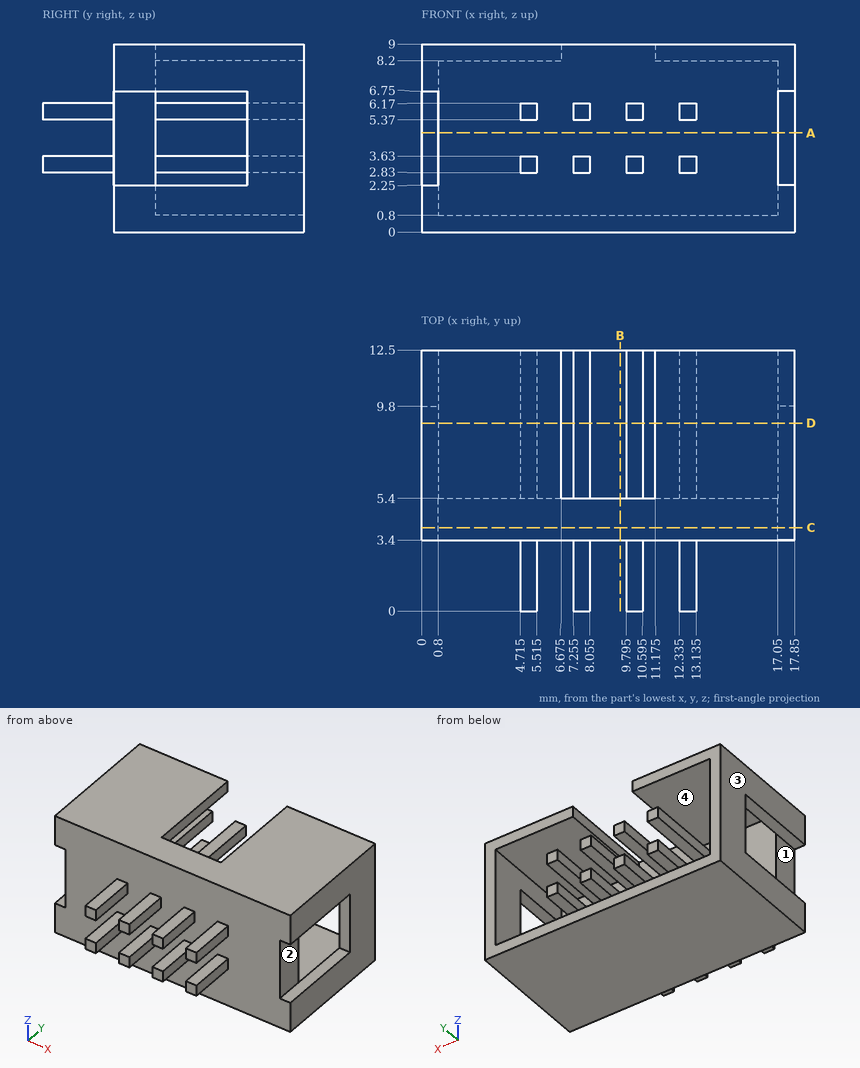
Geometry check sheet. Reference: drawing and pictorial views, mm from the part's lowest x, y, z. A direction names the side the tool comes from. Give positions to 0.01 mm unless a question says otherwise; leave off trailing zeros. Write each loop counter-clockwise with the first axis right and the second up, starting at its lowest first coordinate (ties: lowest second). Pieces come first, ordered by that corner, then holes.
Item 1: Cross-section at C-C (y = 4). Enter the section's corners in (x, z), and give its area (3 significant figures).
Item 2: Access from +Z, -Z, +X, -X, +Y, -Y to the whole of each face (thin tool, end or side, straight path). Record for the marked faces 1, 2, 3 and 4.
Item 3: Cross-section at D-D (y = 9). Count the separate pieces of the cut face and the enclosed holes in it, and give its area (3 significant figures).
Item 4: Cross-section at B-B (x = 9.5). Enter the section's corners in (y, z), and give its area (3 significant figures).
Item 5: Cross-section at A-A (z = 4.75). Enter the section's corners in (x, y), and give its area (3 significant figures).
Item 6: Scan lines: L1, parallel to Z at x = 12.5, y = 11.5; L2, parallel to X at y = 11, z = 3 (3 decimals); L3, parallel to X at y = 6, z = 1.75. Record each from-to range of solid material in increasing order.
Item 7: Gauge pin test, flat ends, axial feed: pin 1 (1 mm diameter, centred on x = 7.5, z = 2, fed in from +Y); pin 2 (0.9 mm diameter, centred on x = 5, y = 1.5, fed in from -Z); pin 3 (0.6 mm diameter, centred on y = 2, z = 6, fed in from +X) (3 decimals). Record the tip position at first contact, or that the pin passes through.
Report:
1. outline: (0, 0) - (17.85, 0) - (17.85, 2.25) - (17.05, 2.25) - (17.05, 6.75) - (17.85, 6.75) - (17.85, 9) - (0, 9) - (0, 6.75) - (0.8, 6.75) - (0.8, 2.25) - (0, 2.25) - close
1. area: 153 mm2
2. face 1: -X, -Y
2. face 2: +X, -Y
2. face 3: +Z, -Z, -X, +Y, -Y
2. face 4: +Y
3. separate pieces: 11
3. enclosed holes: 0
3. area: 34.7 mm2
4. outline: (3.4, 0) - (12.5, 0) - (12.5, 0.8) - (5.4, 0.8) - (5.4, 9) - (3.4, 9) - close
4. area: 23.7 mm2
5. outline: (0, 9.8) - (0.8, 9.8) - (0.8, 12.5) - (0, 12.5) - close; (0.8, 3.4) - (17.05, 3.4) - (17.05, 5.4) - (0.8, 5.4) - close; (17.05, 9.8) - (17.85, 9.8) - (17.85, 12.5) - (17.05, 12.5) - close
5. area: 36.8 mm2
6. L1: z = 0 to 0.8, 2.83 to 3.63, 5.37 to 6.17, 8.2 to 9
6. L2: x = 0 to 0.8, 4.715 to 5.515, 7.255 to 8.055, 9.795 to 10.595, 12.335 to 13.135, 17.05 to 17.85
6. L3: x = 0 to 0.8, 17.05 to 17.85
7. pin 1: stops at y = 5.4
7. pin 2: stops at z = 2.83
7. pin 3: stops at x = 13.135
